Could you check a few things on this model? Use its own coordinates, in mm. Face numbers are marked on the shaded views. A direction names the side the tool comes from. Round coordinates to 2 decimals unless told otherwise and drop trailing zeros. Order: outer loops, then holes, each group sorted by start corner. A loop starts at its lowest first (then second) coordinate and runs counter-clockwise, first axis right, second up. Notation, with made-up numbers: (33.5, 16.25) - (54.5, 16.25) arc R33 ccw to (54.5, 48.25) - close; hole circle Ø2 at (80.5, 9). An arc over 180 degrees is marked (long way). Return JSON: item names as keys, results as strings. Group by question number.
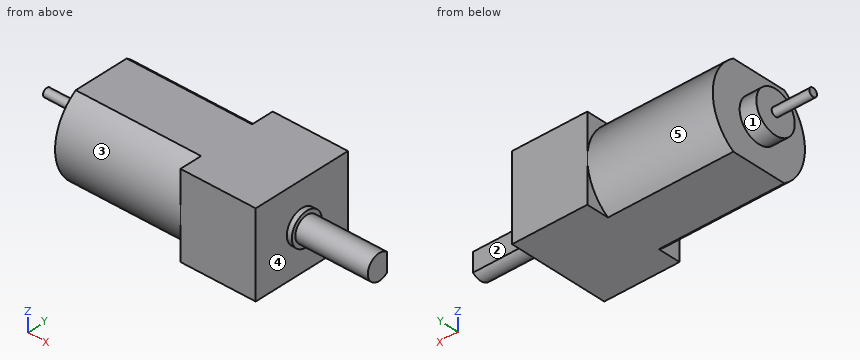
from build123d import *

# Parameters (mm, degrees)
BOSS_EXTRU_1_DEPTH      = 15
ESQUISSE2_R             = 2.5
BOSS_EXTRU_2_DEPTH      = 2
ESQUISSE3_W             = 10
ESQUISSE3_H             = 12
BOSS_EXTRU_3_DEPTH      = 9
ESQUISSE4_R             = 1.95
BOSS_EXTRU_4_DEPTH      = 0.6
ESQUISSE5_R             = 1.5
BOSS_EXTRU_5_DEPTH      = 8.67
ENL_V_START             = -8.67
ENL_V_MAT_EXTRU_1_DEPTH = 8.67
ESQUISSE7_R             = 0.5
BOSS_EXTRU_6_DEPTH      = 4.5


with BuildPart() as part:
    # Esquisse1 → Boss.-Extru.1 (new body)
    with BuildSketch(Plane(origin=(0, 0, 0), x_dir=(0, 0, -1), z_dir=(1, 0, 0))):
        with BuildLine():
            Line((-5, 3.31662479), (-5, -3.31662479))
            ThreePointArc((-5, -3.31662479), (0, -6), (5, -3.31662479))
            Line((5, -3.31662479), (5, 3.31662479))
            ThreePointArc((5, 3.31662479), (0, 6), (-5, 3.31662479))
        make_face()
    extrude(amount=BOSS_EXTRU_1_DEPTH)

    # Esquisse2 → Boss.-Extru.2 (add)
    with BuildSketch(Plane.ZY):
        Circle(ESQUISSE2_R)
    extrude(amount=BOSS_EXTRU_2_DEPTH)

    # Esquisse3 → Boss.-Extru.3 (add)
    with BuildSketch(Plane(origin=(15, 0, 0), x_dir=(0, 0, -1), z_dir=(1, 0, 0))):
        Rectangle(ESQUISSE3_W, ESQUISSE3_H)
    extrude(amount=BOSS_EXTRU_3_DEPTH)

    # Esquisse4 → Boss.-Extru.4 (add)
    with BuildSketch(Plane(origin=(24, 0, 0), x_dir=(0, 0, -1), z_dir=(1, 0, 0))):
        Circle(ESQUISSE4_R)
    extrude(amount=BOSS_EXTRU_4_DEPTH)

    # Esquisse5 → Boss.-Extru.5 (add)
    with BuildSketch(Plane(origin=(24.6, 0, 0), x_dir=(0, 0, -1), z_dir=(1, 0, 0))):
        Circle(ESQUISSE5_R)
    extrude(amount=BOSS_EXTRU_5_DEPTH)

    # Esquisse6 → Enlèv. mat.-Extru.1 (cut)
    with BuildSketch(Plane(origin=(33.27, 0, 0), x_dir=(0, 0, -1), z_dir=(1, 0, 0)).offset(ENL_V_START)):
        with BuildLine():
            Line((-1.118033989, 1), (1.118033989, 1))
            ThreePointArc((1.118033989, 1), (0, 1.5), (-1.118033989, 1))
        make_face()
    extrude(amount=ENL_V_MAT_EXTRU_1_DEPTH, mode=Mode.SUBTRACT)

    # Esquisse7 → Boss.-Extru.6 (add)
    with BuildSketch(Plane.ZY.offset(2)):
        Circle(ESQUISSE7_R)
    extrude(amount=BOSS_EXTRU_6_DEPTH)


solid = part.part
1) I want a section at B-B, the plane y = 4.5. List the corners of the cut face in (x, z) for me.
2) Will these pins go through, and if not, where does the flat tip stop? pin 1 (1.3 mm diameter, centred on y = 4, z = 2.5, fed in from -X); pin 2 (0.7 mm diameter, centred on x = 27.5, z = -0.5, fed in from +Y); pin 3 (3 mm diameter, centred on x = -1, z = -2, fed in from +Y).
3) If I drill on line 1 along X through (y, z) = (-1.5, -2.25); line 2 along Z through (x, y) = (8, -3.5); line 3 along Y through (x, z) = (14, -3.25), over which ranges is the centre line in solid material (lowest first)? Write a range as from..to.
4) For the marked faces 1, 2, 3, 4 and 5, which set-ups out of +Z, -Z, +X, -X, +Y, -Y let a thin tool reach every point of the face, with its end or its side?
5) I want a section at A-A, the plane z = 3.25. List the corners of the cut face in (x, y) for me.
6) I want a section at C-C, the plane x = 30. List the corners of the cut face in (y, z) for me, plus the area to 3 significant figures.
7) I want a section at D-D, the plane x = 4. List the corners of the cut face in (y, z) for me.
Outcome:
{
 "1": {"outline": "(0, -3.97) - (15, -3.97) - (15, -5) - (24, -5) - (24, 5) - (15, 5) - (15, 3.97) - (0, 3.97) - close"},
 "2": {"pin 1": "x = 0", "pin 2": "y = 1", "pin 3": "y = 5.93"},
 "3": {"line 1": "0..24", "line 2": "-4.87..4.87", "line 3": "-5.04..5.04"},
 "4": {"face 1": "-X", "face 2": "+Z, -Z, +X, +Y", "face 3": "-X, -Y", "face 4": "+X", "face 5": "-X, +Y"},
 "5": {"outline": "(0, -5.04) - (15, -5.04) - (15, -6) - (24, -6) - (24, 6) - (15, 6) - (15, 5.04) - (0, 5.04) - close"},
 "6": {"outline": "(1, -1.12) - (1, 1.12) arc R1.5 ccw (long way) to start", "area": "6.29 mm^2"},
 "7": {"outline": "(-3.32, -5) - (3.32, -5) arc R6 ccw to (3.32, 5) - (-3.32, 5) arc R6 ccw to start"}
}
